Build history of the part. All positions in model axes, mm. A direction names the side the tool comes from. Give positions to 0.01 mm unless a question says otherwise; leave off trailing zeros. Order: outer loops, then holes, each group sorted by start corner. A loop starts at its lowest first (then second) coordinate and runs counter-clockwise, first axis right, second up. Notation, with made-up numbers: (81.5, -34) - (100.5, -34) arc R8 cw to (100.5, -21) - close; hole circle Ø9 at (21, 66). An arc over 180 degrees is marked (long way). Answer in a Markdown table with one row per item.
Autodesk Inventor part; units mm, degrees
ref_plane "YZ Plane" through (0, 0, 0) normal (1, 0, 0) x (0, 1, 0)
ref_plane "XZ Plane" through (0, 0, 0) normal (0, 1, 0) x (-1, 0, 0)
ref_plane "XY Plane" through (0, 0, 0) normal (0, 0, 1) x (1, 0, 0)
sketch "スケッチ4" plane through (0, 0, 0) normal (0, 0, 1) x (1, 0, 0)
  arc A0 (0, -3.25) -> (0, 3.25) centre (0, 0) ccw
  circle A1 centre (-7.5, 0) radius 3.25 construction
  arc A2 (12.5, 3.25) -> (12.5, -3.25) centre (12.5, 0) ccw
  arc A3 (20, -3.25) -> (20, 3.25) centre (20, 0) ccw
  arc A4 (12.5, 20) -> (-7.5, 0) centre (12.5, 0) ccw construction
  line L0 (12.5, 3.25) -> (20, 3.25)
  line L1 (20, -3.25) -> (12.5, -3.25)
  arc A5 (12.5, 16.75) -> (12.211, 16.7475) centre (12.5, 0) ccw construction
  circle A6 centre (12.5, 20) radius 3.25 construction
  line L2 (0, 3.25) -> (-3.9317, 3.25)
  line L3 (-7.5, -3.25) -> (-4.25, -3.25) construction
  line L4 (20, 9.25) -> (12.5, 9.25)
  arc A7 (12.5, 9.25) -> (12.5, -9.25) centre (12.5, 0) ccw construction
  line L5 (12.5, -9.25) -> (20, -9.25)
  arc A8 (20, -9.25) -> (20, 9.25) centre (20, 0) ccw
  line L6 (-3.9317, 3.25) -> (-7.5, 3.25) construction
  line L7 (-4.25, 0) -> (-4.25, -3.25) construction
  line L8 (-4.25, -3.25) -> (0, -3.25)
  arc A9 (-3.9317, 3.25) -> (-4.25, 0) centre (12.5, 0) ccw construction
  line L9 (-4.25, -3.25) -> (-4.25, -9.25)
  line L10 (-4.25, -9.25) -> (12.5, -9.25)
  line L11 (20, -9.25) -> (180, -9.25)
  line L12 (180, -9.25) -> (162.8622, 2.75)
  line L13 (162.8622, 2.75) -> (162.8622, -9.25) construction
  arc A10 (11.9, 16.8059) -> (12.211, 16.7475) centre (162.8622, 820.4571) ccw construction
  arc A11 (12.211, 16.7475) -> (162.8622, 2.75) centre (162.8622, 820.4571) ccw
  arc A12 (12.211, 16.7475) -> (-3.9317, 3.25) centre (12.5, 0) ccw
  dimension "d39" = 6.5
  dimension "d40" = 6.5
  dimension "d41" = 6.5
  dimension "d42" = 6.5
  dimension "d43" = 7.5
  dimension "d44" = 7.5
  dimension "d46" = 20
  dimension "d47" = 6
  dimension "d48" = 160
  dimension "d49" = 35
  dimension "d50" = 12
extrude "押し出し3" add sketch "スケッチ4" along normal blind 6
sketch "スケッチ5" plane through (0, 0, 6) normal (0, 0, 1) x (1, 0, 0)
  line L0 (-4.25, -9.25) -> (-5.2687, -8.707)
  line L1 (-7.8081, -11.6738) -> (-5.4042, -14.8709)
  arc A0 (-10.6231, -13.074) -> (-9.2864, -14.5617) centre (-8.6663, -12.6602) ccw
  arc A1 (-5.9588, -15.6467) -> (-5.4042, -14.8709) centre (-5.8038, -15.1714) ccw
  line L2 (-5.9588, -15.6467) -> (-9.2864, -14.5617)
  arc A2 (-10.934, -6.7699) -> (-11.554, -8.6713) centre (-9.5973, -8.2576) ccw
  line L3 (-10.6231, -13.074) -> (-11.554, -8.6713)
  line L4 (-10.934, -6.7699) -> (-7.5867, -3.7623)
  arc A3 (-5.2687, -8.707) -> (-7.8081, -11.6738) centre (-6.2095, -10.4719) ccw
  arc A4 (-6.25, -3.25) -> (-7.5867, -3.7623) centre (-6.25, -5.25) ccw
  line L5 (-6.25, -3.25) -> (-4.25, -3.25)
  line L6 (-4.25, -3.25) -> (-4.25, -9.25)
  line L7 (-4.25, -3.25) -> (-4.25, -9.25)
  line L8 (0, -3.25) -> (-4.25, -3.25)
  point P0 (0, 0)
  dimension "d54" = 2
  dimension "d55" = 2
  dimension "d56" = 4.5
  dimension "d57" = 2
  dimension "d58" = 4.5
  dimension "d59" = 2
  dimension "d60" = 3.5
  dimension "d61" = 0.5
  dimension "d62" = 4
  dimension "d63" = 2
  dimension "d65" = 25
  dimension "d66" = 35
  dimension "d67" = 120
  dimension "d68" = 120
  dimension "d97" = 1.1544
  dimension "d98" = 61.94
extrude "押し出し4" add sketch "スケッチ5" against normal blind 6
fillet "フィレット2" radius 1 2 edges at (162.8622, 2.75, 3) (180, -9.25, 3)
sketch "スケッチ6" plane through (0, 0, 6) normal (0, 0, 1) x (1, 0, 0)
  arc A0 (12.211, 16.7475) -> (162.5472, 2.7501) centre (162.8622, 820.4571) ccw
  line L0 (-4.25, -9.25) -> (176.8284, -9.25)
  arc A1 (20, -3.25) -> (20, 3.25) centre (20, 0) ccw
  line L1 (12.5, 3.25) -> (20, 3.25)
  line L2 (20, -3.25) -> (12.5, -3.25)
  line L3 (177.402, -7.4308) -> (163.1204, 2.5692)
  arc A2 (176.8284, -9.25) -> (177.402, -7.4308) centre (176.8284, -8.25) ccw
  arc A3 (163.1204, 2.5692) -> (162.5472, 2.7501) centre (162.5468, 1.7501) ccw
  line L4 (163.3443, -1.2499) -> (170.4852, -6.25)
  arc A4 (12.211, 10.7475) -> (26.5915, 8.9414) centre (206.3266, 1498.1342) ccw construction
  line L5 (12.5, -2.25) -> (28.858, -2.6642) construction
  line L6 (163.3443, -1.2499) -> (163.3443, 2.7501)
  line L7 (12.5, 9.25) -> (20, 9.25) construction
  arc A5 (20, -9.25) -> (28.858, -2.6642) centre (20, 0) ccw construction
  line L8 (20, -9.25) -> (12.5, -9.25)
  arc A6 (26.5915, 8.9414) -> (25.8403, 7.1731) centre (26.4717, 7.9486) ccw
  arc A7 (28.858, -2.6642) -> (25.8403, 7.1731) centre (20, 0) ccw
  line L9 (28.858, -2.6642) -> (170.4852, -6.25)
  arc A8 (26.5915, 8.9414) -> (163.3443, -1.2499) centre (206.3266, 1498.1342) ccw
  arc A9 (25.8403, 7.1731) -> (20, 9.25) centre (20, 0) ccw construction
  point P0 (0, 0)
  dimension "d73" = 3
  dimension "d74" = 6
  dimension "d75" = 7
  dimension "d76" = 4
  dimension "d77" = 3
  dimension "d80" = 1500
  dimension "d81" = 6
  dimension "d82" = 2
extrude "押し出し5" cut sketch "スケッチ6" against normal blind 6
fillet "フィレット3" radius 1 3 edges at (163.3443, -1.2499, 3) (28.858, -2.6642, 3) (170.4852, -6.25, 3)
sketch "スケッチ8" plane through (0, 0, 6) normal (0, 0, 1) x (1, 0, 0)
  arc A0 (26.5915, 8.9414) -> (163.0449, -1.2412) centre (206.3266, 1498.1342) ccw
  arc A1 (163.5897, -1.4217) -> (163.0449, -1.2412) centre (163.0161, -2.2408) ccw
  line L0 (163.5897, -1.4217) -> (167.7677, -4.3472)
  arc A2 (167.1689, -6.166) -> (167.7677, -4.3472) centre (167.1942, -5.1664) ccw
  line L1 (167.1689, -6.166) -> (30.0835, -2.6952)
  arc A3 (29.1226, -1.5301) -> (30.0835, -2.6952) centre (30.1088, -1.6955) ccw
  arc A4 (29.1226, -1.5301) -> (25.8403, 7.1731) centre (20, 0) ccw
  arc A5 (26.5915, 8.9414) -> (25.8403, 7.1731) centre (26.4717, 7.9486) ccw
  arc A6 (176.8284, -9.25) -> (177.402, -7.4308) centre (176.8284, -8.25) ccw
  line L2 (177.402, -7.4308) -> (163.1204, 2.5692)
  arc A7 (163.1204, 2.5692) -> (162.5472, 2.7501) centre (162.5468, 1.7501) ccw
  arc A8 (12.211, 16.7475) -> (162.5472, 2.7501) centre (162.8622, 820.4571) ccw
  arc A9 (12.211, 16.7475) -> (-3.9317, 3.25) centre (12.5, 0) ccw
  line L3 (-3.9317, 3.25) -> (0, 3.25)
  arc A10 (0, -3.25) -> (0, 3.25) centre (0, 0) ccw
  arc A11 (-6.25, -3.25) -> (-7.5867, -3.7623) centre (-6.25, -5.25) ccw
  line L4 (-7.5867, -3.7623) -> (-10.934, -6.7699)
  arc A12 (-10.934, -6.7699) -> (-11.554, -8.6713) centre (-9.5973, -8.2576) ccw
  line L5 (-11.554, -8.6713) -> (-10.6231, -13.074)
  arc A13 (-10.6231, -13.074) -> (-9.2864, -14.5617) centre (-8.6663, -12.6602) ccw
  line L6 (-9.2864, -14.5617) -> (-5.9588, -15.6467)
  arc A14 (-5.9588, -15.6467) -> (-5.4042, -14.8709) centre (-5.8038, -15.1714) ccw
  line L7 (-5.4042, -14.8709) -> (-7.8081, -11.6738)
  arc A15 (-5.2687, -8.707) -> (-7.8081, -11.6738) centre (-6.2095, -10.4719) ccw
  line L8 (-5.2687, -8.707) -> (-4.25, -9.25)
  line L9 (-4.25, -9.25) -> (176.8284, -9.25)
  line L10 (12.5, 3.25) -> (20, 3.25)
  arc A16 (20, -3.25) -> (20, 3.25) centre (20, 0) ccw
  line L11 (20, -3.25) -> (12.5, -3.25)
  arc A17 (12.5, 3.25) -> (12.5, -3.25) centre (12.5, 0) ccw
  line L12 (0, -3.25) -> (-6.25, -3.25)
extrude "押し出し6" add sketch "スケッチ8" against normal blind 0.7 contours A0 A1 L0 A2 L1 A3 A4 A5
fillet "フィレット5" radius 1 1 edges at (-3.9317, 3.25, 3)
equation "\"d44\" = d43"
properties part number "ウイング1" material "ポリカーボネート、クリア"
1. Cut at A-A on x = 124.5. Write the cut outline in (y, z).
Check result:
| item | result |
|---|---|
| outline | (-9.25, 0) - (-5.09, 0) - (-5.09, 5.3) - (0.37, 5.3) - (0.37, 0) - (3.65, 0) - (3.65, 6) - (-9.25, 6) - close |
2. Cut at D-D on y = 14. Write the cut outline in (x, z).
Check result:
| item | result |
|---|---|
| outline | (3.3, 0) - (27.69, 0) - (27.69, 6) - (3.3, 6) - close |
3. Which spindle directions (+Z, -Z, +X, -X, +Y, -Y) get a long thin tool onto all of the face, cutting with end or side? Do faces 4 (the face through (-3, -3.25, 3)), 5 (the face through (28.68, 3.2, 2.69)), 6 (the face through (16, 3.25, 3)). Say none if no direction does.
Check result:
| item | result |
|---|---|
| face 4 | +Z, -Z, -X |
| face 5 | -Z |
| face 6 | +Z, -Z |
4. Probe line 1 (Y direction, x = 90, z = 3.6); line 2 (Y direction, x = 17, z = 0.45); line 3 (Z direction, x = 84.5, y = -3.5). List the from-to ranges inside material, lowest first.
Check result:
| item | result |
|---|---|
| line 1 | y = -9.25 to -4.21, 2.65 to 6 |
| line 2 | y = -9.25 to -3.25, 3.25 to 15.86 |
| line 3 | z = 5.3 to 6 |
5. Cut at B-B on z = 3.05. Count the separate pieces of the cut face and the enclosed holes in it, and give its area (3 significant figures).
Check result:
| item | result |
|---|---|
| separate pieces | 1 |
| enclosed holes | 2 |
| area | 1,930 mm² |
6. Two-plate mould, pull along X, no slides. Class faces 1 (the face through (80, 0, 5.3)), 2 (the face through (82, 1, 6)), 3 (the face through (-7.6, -15.11, 3.04)): +X half, -X half, draft (parallel to the pull), parting line (faces both ways), or undercut.
Check result:
| item | result |
|---|---|
| face 1 | undercut |
| face 2 | draft |
| face 3 | -X half |
7. Cut at C-C on x = 100.5. Write the cut outline in (y, z), and give its area (3 significant figures).
Check result:
| item | result |
|---|---|
| outline | (-9.25, 0) - (-4.48, 0) - (-4.48, 5.3) - (1.87, 5.3) - (1.87, 0) - (5.13, 0) - (5.13, 6) - (-9.25, 6) - close |
| area | 52.6 mm² |
8. Drop flat-ended pins along their axis: P1, Ø1.8, axis at x = 17.5, z = 2.5, coming from the +Y side; P2, Ø2, axis at x = 95, z = 1.5, coming from the -Y side; P3, Ø16.5, axis at x = 86, y = 0, coming from the -Z side. Give the stop position or say it passes through.
Check result:
| item | result |
|---|---|
| P1 | stops at y = 15.94 |
| P2 | stops at y = -9.25 |
| P3 | stops at z = 0 |
